Input: part model. Units: mm. Frame: model coordinates. A direction names the side the tool comes from. Round coordinates to 2 decimals unless told otherwise and drop trailing zeros. Loops run counter-clockwise (first coordinate to the right, second up) from the corner with the lowest first, then second, coordinate; pieces in that order, holes last. Notation, with made-up numbers: M 21,-12.5 L 57,-12.5 A31 cw 57,22.5 Z; hole C -27,48 d6. An arc over 180 degrees is marked long. Put each result on its own line as item: value. Start each with the question number.
1) Line query: probe 1 along X at (y, z) = (4.5, 0) (1 decimal); probe 2 along Z at (x, y) = (0, 6.25); probe 3 along Y at (x, z) = (-8, 1.5). Output: solid intervals per line, ascending.
2) Section D-D on y = 8. Output: boundary loops of the cut face in (x, z) (1 decimal).
3) Reachability of faces 1 (the face through (4, 0, -6)), 2 (the face through (0, 9, 12.7)) from +Z, -Z, +X, -X, +Y, -Y: full face, straight path, thin tool, end or side. Return the list, or none.
4) Section B-B on y = -3.5. Output: boundary loops of the cut face in (x, z) (3 decimals), plus the area to 3 significant figures.
5) Pin query (flat end, axial travel): pin 1 (6 mm diameter, centred on x = 3, z = -2, fed in from -Y); pin 2 (7.5 mm diameter, centred on x = 0, z = 0, fed in from -Y) (3 decimals); pin 3 (12 mm diameter, centred on y = -3, z = 3.5, fed in from +X) (3 decimals). Return the tip coordinate at first contact, or that it passes through.
6) Draft query along Z for faces 3 (the face through (-12.847, -4.696, -0.954)), 4 (the face through (-1.363, 4.696, 6.137)), 5 (the face through (-16, -9.525, 0)), 6 (the face through (0, 9.525, 0)). Return one class per face: +Z half, -Z half, draft (parallel to the pull), parting line (faces both ways), or undercut.
from build123d import *

# Parameters (mm, degrees)
SKETCH1_W           = 41.91
SKETCH1_H           = 25.4
BOSS_EXTRUDE1_DEPTH = 19.05
SKETCH1_4_R         = 6.2865
CUT_EXTRUDE1_DEPTH  = 9.525
SKETCH1_5_R         = 3.175
BOSS_EXTRUDE2_DEPTH = 9.525


with BuildPart() as part:
    # Sketch1 → Boss-Extrude1 (new body)
    with BuildSketch(Plane(origin=(0, 0, 0), x_dir=(1, 0, 0), z_dir=(0, 1, 0))):
        Rectangle(SKETCH1_W, SKETCH1_H)
    extrude(amount=BOSS_EXTRUDE1_DEPTH)

    # Sketch1<4> → Cut-Extrude1 (cut)
    with BuildSketch(Plane(origin=(0, 0, 0), x_dir=(1, 0, 0), z_dir=(0, 1, 0))):
        Circle(SKETCH1_4_R)
    extrude(amount=CUT_EXTRUDE1_DEPTH, mode=Mode.SUBTRACT)

    # Sketch1<5> → Boss-Extrude2 (add)
    with BuildSketch(Plane(origin=(0, 0, 0), x_dir=(1, 0, 0), z_dir=(0, 1, 0))):
        with Locations((-15.875, 0)):
            Circle(SKETCH1_5_R)
        with Locations((15.875, 0)):
            Circle(SKETCH1_5_R)
    extrude(amount=-BOSS_EXTRUDE2_DEPTH)


solid = part.part
Geometry results:
1. probe 1: x = -21 to -6.3, 6.3 to 21
1. probe 2: z = -12.7 to -6.29, 6.29 to 12.7
1. probe 3: y = 0 to 19.05
2. outline: M -21,-12.7 L 21,-12.7 L 21,12.7 L -21,12.7 Z; hole C 0,0 d12.6
3. face 1: -Y
3. face 2: +Z, +X, -X, +Y, -Y
4. outline: C -15.875,0 d6.35; C 15.875,0 d6.35
4. area: 63.3 mm²
5. pin 1: stops at y = 0
5. pin 2: stops at y = 9.525
5. pin 3: stops at x = 20.955
6. face 3: parting line
6. face 4: undercut
6. face 5: draft
6. face 6: undercut
